```python
from build123d import *

# Parameters (mm, degrees)
BOSS_EXTRUDE1_DEPTH = 100
SKETCH2_R           = 3
CUT_EXTRUDE1_DEPTH  = 10


with BuildPart() as part:
    # Sketch1 → Boss-Extrude1 (new body)
    with BuildSketch(Plane(origin=(0, 0, 0), x_dir=(1, 0, 0), z_dir=(0, 1, 0))):
        Polygon((0, 0), (0, 1), (20, 1), (20, 21), (21, 21), (21, 0), align=None)
    extrude(amount=BOSS_EXTRUDE1_DEPTH)

    # Sketch2 → Cut-Extrude1 (cut)
    with BuildSketch(Plane(origin=(0, 0, -1), x_dir=(-1, 0, 0), z_dir=(0, 0, -1))):
        with Locations((-10, 15)):
            Circle(SKETCH2_R)
        with Locations((-10, 50)):
            Circle(SKETCH2_R)
        with Locations((-10, 85)):
            Circle(SKETCH2_R)
    extrude(amount=-CUT_EXTRUDE1_DEPTH, mode=Mode.SUBTRACT)


solid = part.part
```
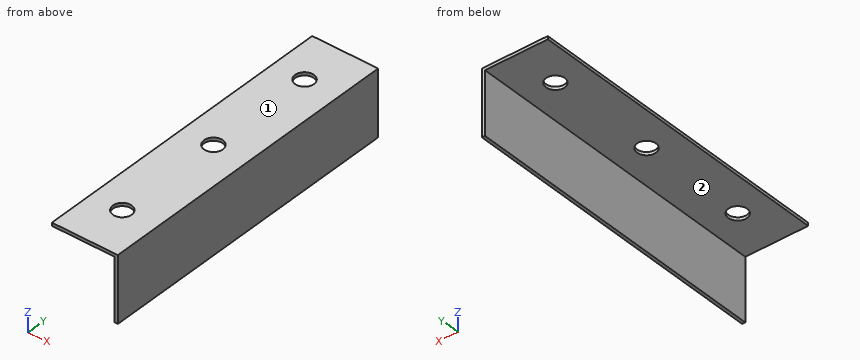
Verification items for the finished model (mm, model axes). Face numbers are marked on the shaded views. A direction names the side the tool comes from. Coordinates: 2 decimals unless noted, no trailing zeros. Loops run counter-clockwise (first coordinate to the right, second up) from the corner with the lowest first, then second, coordinate; pieces in that order, holes last. Notation, with made-up numbers: (69, 47.5) - (88, 47.5) arc R10 cw to (88, 66.5) - close; hole circle Ø2 at (3, 85.25). An arc over 180 degrees is marked (long way). Put each result on its own line as item: value.
Item 1: Gauge pin test, flat ends, axial feed: pin 1 Ø6 at (x, y) = (6, 49.5) entering from -Z; pin 2 Ø8 at (x, y) = (4, 31) entering from +Z. Record the tip position at first contact, or that the pin passes through.
Conclusion:
pin 1: stops at z = -1
pin 2: stops at z = 0
Item 2: Section check A-A (y = 85). Enter the section's corners in (x, z), then the cut area to 3 significant figures.
Conclusion:
outline: (0, -1) - (7, -1) - (7, 0) - (0, 0) - close; (13, -1) - (20, -1) - (20, -21) - (21, -21) - (21, 0) - (13, 0) - close
area: 35.0 mm2
Item 3: Section check D-D (z = -7.25). Enter the section's corners in (x, y).
Conclusion:
outline: (20, 0) - (21, 0) - (21, 100) - (20, 100) - close
Item 4: Scan lines: line 1 along Y through (x, z) = (10, -0.3); line 2 along X through (y, z) = (74, -14); line 3 along Z through (x, y) = (13.5, 34). Record each from-to range of solid material in increasing order.
Conclusion:
line 1: y = 0 to 12, 18 to 47, 53 to 82, 88 to 100
line 2: x = 20 to 21
line 3: z = -1 to 0
Item 5: Section check C-C (y = 22). Enter the section's corners in (x, z).
Conclusion:
outline: (0, -1) - (20, -1) - (20, -21) - (21, -21) - (21, 0) - (0, 0) - close
Item 6: Set-up check for the marked faces 1 and 2: record each of +Z, -Z, +X, -X, +Y, -Y from which the full face is reachable in a straight line by a thin tool's end or side.
Conclusion:
face 1: +Z, +X, -X, +Y, -Y
face 2: -Z, -X, +Y, -Y
Item 7: Section check B-B (x = 10). Enter the section's corners in (y, z), then the cut area to 3 significant figures.
Conclusion:
outline: (0, -1) - (12, -1) - (12, 0) - (0, 0) - close; (18, -1) - (47, -1) - (47, 0) - (18, 0) - close; (53, -1) - (82, -1) - (82, 0) - (53, 0) - close; (88, -1) - (100, -1) - (100, 0) - (88, 0) - close
area: 82.0 mm2
